Verification items for this drawing (mm, ordinates from the low corner). A direction names the side the tool comes from. Give positions to 0.01 mm unless a question says otherwise; leave off trailing zeros. Loops run counter-clockwise (first coordinate to the right, second up) from the corner with the lowest first, then second, coordinate; pieces in that order, holes last. Notation, with made-up numbers: (5, 13) -> (10, 13) arc R21 ccw to (10, 17) -> close; hole circle Ø7 at (-37.5, -35.5). An arc over 180 degrees is marked (long way). Use one line per item in the form item = value. Start each with the question number.
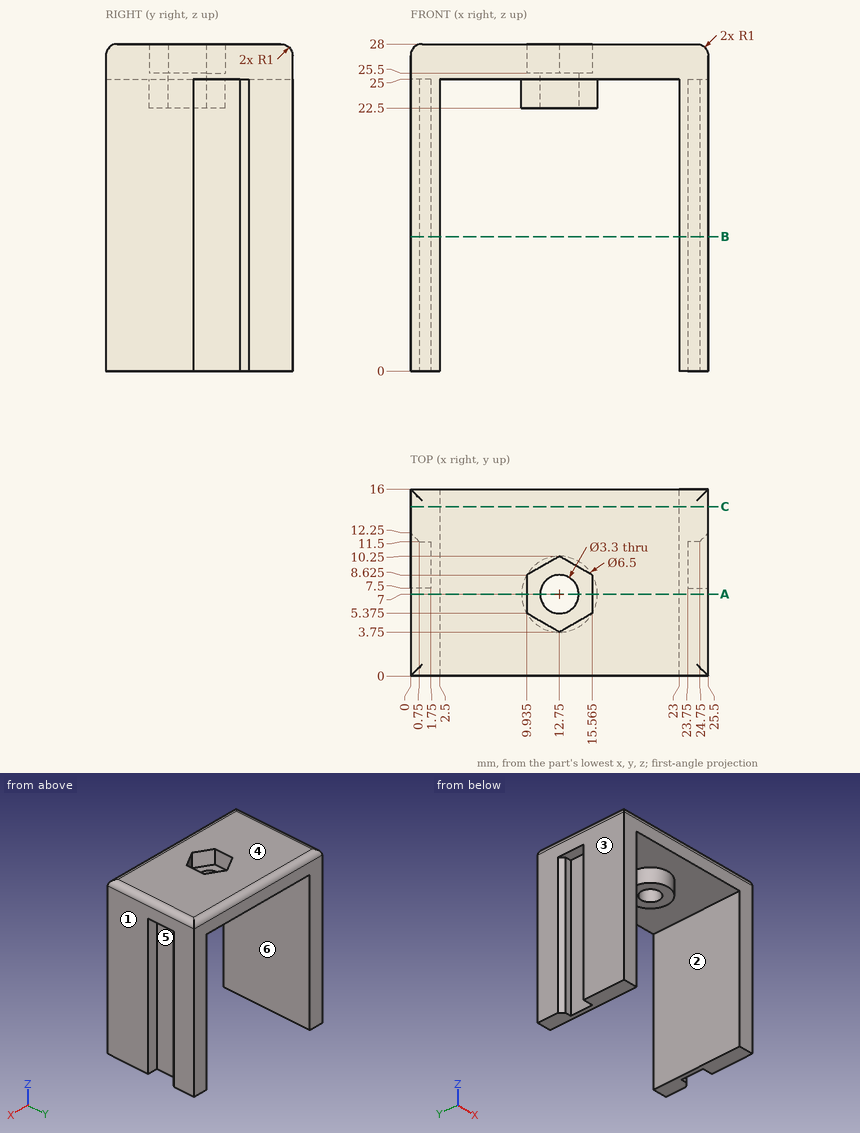
Item 1: Draft check along X on the marked faces 3, 4, 5 and 6. Enter one of: +X half, -X half, draft (parallel to the pull), parting line (faces both ways), or undercut.
Item 2: Gauge pin test, flat ends, axial feed: pin 1 Ø4.5 at (x, y) = (12.75, 7) entering from -Z; pin 2 Ø1.5 at (x, y) = (22, 13) entering from -Z. Record the tip position at first contact, or that the pin passes through.
Item 3: Sectioned sample at A-A, the plane y = 7. Enter the section's corners in (x, z) (1 decimal).
Item 4: Sectioned sample at C-C, the plane y = 14.5. Enter the section's corners in (x, z), and give its area (3 significant figures).
Item 5: Tool access check on the marked faces 1 and 2. Record the directions out of +Z, -Z, +X, -X, +Y, -Y that give a thin tool (end or side, any length) a straight path to the whole face; none if there is none.
Item 6: Material ranges on line 1 (X direction, y = 3, z = 17.25); line 2 (Y direction, x = 1.5, z = 20); line 3 (X direction, y = 8.5, z = 13.5), recorded low to high.
Item 7: Sectioned sample at B-B, the plane z = 11.5. Enter the section's corners in (x, y).
Outcome:
q1.face_3 = -X half
q1.face_4 = draft
q1.face_5 = +X half
q1.face_6 = undercut
q2.pin_1 = 22.5
q2.pin_2 = 25
q3.outline = (0, 0) -> (2.5, 0) -> (2.5, 25) -> (9.5, 25) -> (9.5, 22.5) -> (11.1, 22.5) -> (11.1, 25.5) -> (9.9, 25.5) -> (9.9, 28) -> (1, 28) arc R1 ccw to (0, 27) -> close; (14.4, 22.5) -> (16, 22.5) -> (16, 25) -> (23, 25) -> (23, 0) -> (25.5, 0) -> (25.5, 27) arc R1 ccw to (24.5, 28) -> (15.6, 28) -> (15.6, 25.5) -> (14.4, 25.5) -> close
q4.outline = (0, 0) -> (2.5, 0) -> (2.5, 25) -> (23, 25) -> (23, 0) -> (25.5, 0) -> (25.5, 27) arc R1 ccw to (24.5, 28) -> (1, 28) arc R1 ccw to (0, 27) -> close
q4.area = 201 mm^2
q5.face_1 = +Z, -Z, +X, +Y, -Y
q5.face_2 = -Z, +Y, -Y
q6.line_1 = 0 to 2.5, 23 to 25.5
q6.line_2 = 0 to 7.5, 11.5 to 16
q6.line_3 = 1.75 to 2.5, 23 to 23.75
q7.outline = (0, 0) -> (2.5, 0) -> (2.5, 16) -> (0, 16) -> (0, 12.25) -> (0.75, 11.5) -> (1.75, 11.5) -> (1.75, 7.5) -> (0, 7.5) -> close; (23, 0) -> (25.5, 0) -> (25.5, 7.5) -> (23.75, 7.5) -> (23.75, 11.5) -> (24.75, 11.5) -> (25.5, 12.25) -> (25.5, 16) -> (23, 16) -> close
